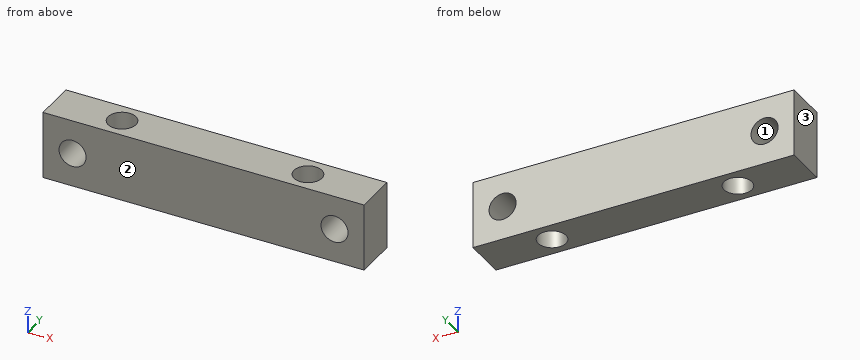
```python
from build123d import *

# Parameters (mm, degrees)
CROQUIS1_W                          = 38
CROQUIS1_H                          = 5
SALIENTE_EXTRUIR1_DEPTH             = 8
DI_METRO_DE_TALADRO_3_2_3_2_1_D     = 3.2
DI_METRO_DE_TALADRO_3_2_3_2_1_DEPTH = 12
DI_METRO_DE_TALADRO_3_2_3_2_1_TIP   = 0.96137699
TALADRO_ROSCADO_M41_D               = 3.3
TALADRO_ROSCADO_M41_DEPTH           = 8


with BuildPart() as part:
    # Croquis1 → Saliente-Extruir1 (new body)
    with BuildSketch(Plane.XY):
        with Locations((19, 2.5)):
            Rectangle(CROQUIS1_W, CROQUIS1_H)
    extrude(amount=SALIENTE_EXTRUIR1_DEPTH)

    # Diámetro de taladro Ø3.2 (3.2)1
    with Locations(Plane(origin=(3.5, 5, 4), x_dir=(0, 0, 1), z_dir=(0, 1, 0))):
        with Locations((0, 0), (0, 31)):
            Hole(DI_METRO_DE_TALADRO_3_2_3_2_1_D / 2, depth=DI_METRO_DE_TALADRO_3_2_3_2_1_DEPTH)
            with Locations((0, 0, -(DI_METRO_DE_TALADRO_3_2_3_2_1_DEPTH + DI_METRO_DE_TALADRO_3_2_3_2_1_TIP / 2))):  # 118° drill point
                Cone(0, DI_METRO_DE_TALADRO_3_2_3_2_1_D / 2, DI_METRO_DE_TALADRO_3_2_3_2_1_TIP, mode=Mode.SUBTRACT)

    # Taladro roscado M41
    with Locations(Plane(origin=(8, 2.5, 0), x_dir=(-1, 0, 0), z_dir=(0, 0, -1))):
        with Locations((0, 0), (-22, 0)):
            Hole(TALADRO_ROSCADO_M41_D / 2, depth=TALADRO_ROSCADO_M41_DEPTH)


solid = part.part
```
Geometry check sheet. Reference: the model listing, model coordinates, mm. Face numbers are marked on the shaded views. Give positions to 0.01 mm unless a question says otherwise; leave off trailing zeros. Write each loop counter-clockwise with the first axis right and the second up, starting at its lowest first coordinate (ties: lowest second). Pieces come first, ordered by that corner, then holes. Notation, with made-up numbers: (48, -13.5) - (62, -13.5) arc R10 ccw to (62, -9.5) - close; hole circle Ø4 at (89.25, 38.25). An arc over 180 degrees is marked (long way). Use a Markdown table: item, result.
Q1. Section check B-B, the plane z = 4. Enter the section's corners in (x, y).
Computed:
| item | result |
|---|---|
| outline | (0, 0) - (1.9, 0) - (1.9, 5) - (0, 5) - close; (5.1, 0) - (32.9, 0) - (32.9, 5) - (5.1, 5) - close; (36.1, 0) - (38, 0) - (38, 5) - (36.1, 5) - close; hole circle Ø3.3 at (8, 2.5); hole circle Ø3.3 at (30, 2.5) |
Q2. Section check A-A, the plane y = 2.5. Enter the section's corners in (x, z), then the cut area to 3 significant figures.
Computed:
| item | result |
|---|---|
| outline | (0, 0) - (6.35, 0) - (6.35, 8) - (0, 8) - close; (9.65, 0) - (28.35, 0) - (28.35, 8) - (9.65, 8) - close; (31.65, 0) - (38, 0) - (38, 8) - (31.65, 8) - close; hole circle Ø3.2 at (3.5, 4); hole circle Ø3.2 at (34.5, 4) |
| area | 235 mm² |
Q3. Section check D-D, the plane z = 6. Enter the section's corners in (x, y).
Computed:
| item | result |
|---|---|
| outline | (0, 0) - (38, 0) - (38, 5) - (0, 5) - close; hole circle Ø3.3 at (8, 2.5); hole circle Ø3.3 at (30, 2.5) |
Q4. Section check C-C, the plane x = 30. Enter the section's corners in (y, z), then the cut area to 3 significant figures.
Computed:
| item | result |
|---|---|
| outline | (0, 0) - (0.85, 0) - (0.85, 8) - (0, 8) - close; (4.15, 0) - (5, 0) - (5, 8) - (4.15, 8) - close |
| area | 13.6 mm² |
Q5. Draft check along X on the marked faces 1, 2 and 3. Enter one of: pulls with the +X half, pulls with the -X half, needs draft (parallel to the pull), parting line crosses it, or undercut.
Computed:
| item | result |
|---|---|
| face 1 | undercut |
| face 2 | needs draft |
| face 3 | pulls with the -X half |
Q6. Thickness scan on L1, parallel to X at y = 1.7, z = 7.5; L2, parallel to Y at x = 30, z = 5.75; L3, parallel to X at y = 1, z = 6.5. Record the ranges inside material, lowest first. Write a range as [from, to].
Computed:
| item | result |
|---|---|
| L1 | x = [0, 6.56], [9.44, 28.56], [31.44, 38] |
| L2 | y = [0, 0.85], [4.15, 5] |
| L3 | x = [0, 7.31], [8.69, 29.31], [30.69, 38] |
